Model file for the job. Use its own axes, mm. A direction names the side the tool comes from. Coordinates: 2 decimals unless noted, no trailing zeros. Order: outer loops, then holes, each group sorted by start corner. A loop starts at its lowest first (then second) coordinate and runs counter-clockwise, first axis right, second up.
from build123d import *
from OCP.BRepFilletAPI import BRepFilletAPI_MakeChamfer

# Parameters (mm, degrees)
ESQUISSE1_W           = 12
ESQUISSE1_H           = 12
BOSS_EXTRU_1_DEPTH    = 6.3
ESQUISSE2_R           = 3.4
BOSS_EXTRU_2_DEPTH    = 5
ESQUISSE5_R           = 1.8
BOSS_EXTRU_5_DEPTH    = 0.5
ESQUISSE3_R           = 3
BOSS_EXTRU_3_DEPTH    = 2.5
BOSS_EXTRU_6_START    = 2.5
BOSS_EXTRU_6_DEPTH    = 7
ESQUISSE4_W           = 1
ESQUISSE4_H           = 0.25
BOSS_EXTRU_4_DEPTH    = 3.8
CHANFREIN1_SIZE       = 0.5
CONG_1_R              = 1
CHANFREIN2_SIZE       = 0.3
CHANFREIN2_SIZE2      = 0.519615242
BOSS_EXTRU_7_START    = -1.2
BOSS_EXTRU_7_DEPTH    = 2
CONG_2_R              = 1
CONG_2_OF_SYM_TRIE1_R = 1


with BuildPart() as part:
    # Esquisse1 → Boss.-Extru.1 (new body)
    with BuildSketch(Plane.XY):
        Rectangle(ESQUISSE1_W, ESQUISSE1_H)
    extrude(amount=BOSS_EXTRU_1_DEPTH)

    # Esquisse2 → Boss.-Extru.2 (add)
    with BuildSketch(Plane.XY.offset(6.3)):
        Circle(ESQUISSE2_R)
    extrude(amount=BOSS_EXTRU_2_DEPTH)

    # Esquisse5 → Boss.-Extru.5 (add)
    with BuildSketch(Plane.XY.offset(11.3)):
        Circle(ESQUISSE5_R)
    extrude(amount=BOSS_EXTRU_5_DEPTH)

    # Esquisse3 → Boss.-Extru.3 (add)
    with BuildSketch(Plane.XY.offset(11.8)):
        Circle(ESQUISSE3_R)
    extrude(amount=BOSS_EXTRU_3_DEPTH)

    # Esquisse3<4> → Boss.-Extru.6 (add)
    with BuildSketch(Plane.XY.offset(11.8).offset(BOSS_EXTRU_6_START)):
        with BuildLine():
            Line((1.5, 0.994987437), (1.5, 2.598076211))
            ThreePointArc((1.5, 2.598076211), (-3, 0), (1.5, -2.598076211))
            Line((1.5, -2.598076211), (1.5, -0.994987437))
            ThreePointArc((1.5, -0.994987437), (-1.8, 0), (1.5, 0.994987437))
        make_face()
        with BuildLine():
            Line((1.5, -0.994987437), (1.5, 0.994987437))
            ThreePointArc((1.5, 0.994987437), (-1.8, 0), (1.5, -0.994987437))
        make_face()
    extrude(amount=BOSS_EXTRU_6_DEPTH)

    # Esquisse4 → Boss.-Extru.4 (add)
    with BuildSketch(Plane.XZ.offset(6)):
        with Locations((0, 3.5)):
            Rectangle(ESQUISSE4_W, ESQUISSE4_H)
        with Locations((2.35, 3.5)):
            Rectangle(ESQUISSE4_W, ESQUISSE4_H)
        with Locations((-2.35, 3.5)):
            Rectangle(ESQUISSE4_W, ESQUISSE4_H)
        with Locations((-2.35, 1)):
            Rectangle(ESQUISSE4_W, ESQUISSE4_H)
        with Locations((2.35, 1)):
            Rectangle(ESQUISSE4_W, ESQUISSE4_H)
    extrude(amount=BOSS_EXTRU_4_DEPTH)

    # Chanfrein1
    chanfrein1_edges = [part.edges().sort_by_distance(p)[0] for p in [
        (1.5, 0, 21.3),
        (-3, 0, 21.3),
    ]]
    chamfer(chanfrein1_edges, length=CHANFREIN1_SIZE)

    # Congé1
    cong_1_edges = [part.edges().sort_by_distance(p)[0] for p in [
        (6, -6, 3.15),
        (-6, -6, 3.15),
        (-6, 6, 3.15),
        (6, 6, 3.15),
    ]]
    fillet(cong_1_edges, radius=CONG_1_R)

    # Chanfrein2: one chamfer whose edges measure the first distance from different faces: ONE call of the kernel's chamfer builder (chamfer() names one face for all edges)
    chanfrein2_edges_1 = [part.edges().sort_by_distance(p)[0] for p in [
        (0.5, -6, 3.5),
    ]]
    chanfrein2_side_1 = [part.faces().sort_by_distance(p)[0] for p in [
        (0.5, -7.9, 3.5),
    ]]
    chanfrein2_edges_2 = [part.edges().sort_by_distance(p)[0] for p in [
        (-0.5, -6, 3.5),
    ]]
    chanfrein2_side_2 = [part.faces().sort_by_distance(p)[0] for p in [
        (-0.5, -7.9, 3.5),
    ]]
    chanfrein2_edges_3 = [part.edges().sort_by_distance(p)[0] for p in [
        (0.5, -9.8, 3.5),
        (-0.5, -9.8, 3.5),
    ]]
    chanfrein2_side_3 = [part.faces().sort_by_distance(p)[0] for p in [
        (0, -9.8, 3.5),
    ]]
    chanfrein2_edges_4 = [part.edges().sort_by_distance(p)[0] for p in [
        (2.85, -6, 3.5),
    ]]
    chanfrein2_side_4 = [part.faces().sort_by_distance(p)[0] for p in [
        (2.85, -7.9, 3.5),
    ]]
    chanfrein2_edges_5 = [part.edges().sort_by_distance(p)[0] for p in [
        (1.85, -6, 3.5),
    ]]
    chanfrein2_side_5 = [part.faces().sort_by_distance(p)[0] for p in [
        (1.85, -7.9, 3.5),
    ]]
    chanfrein2_edges_6 = [part.edges().sort_by_distance(p)[0] for p in [
        (2.85, -9.8, 3.5),
        (1.85, -9.8, 3.5),
    ]]
    chanfrein2_side_6 = [part.faces().sort_by_distance(p)[0] for p in [
        (2.35, -9.8, 3.5),
    ]]
    chanfrein2_edges_7 = [part.edges().sort_by_distance(p)[0] for p in [
        (-1.85, -6, 3.5),
    ]]
    chanfrein2_side_7 = [part.faces().sort_by_distance(p)[0] for p in [
        (-1.85, -7.9, 3.5),
    ]]
    chanfrein2_edges_8 = [part.edges().sort_by_distance(p)[0] for p in [
        (-2.85, -6, 3.5),
    ]]
    chanfrein2_side_8 = [part.faces().sort_by_distance(p)[0] for p in [
        (-2.85, -7.9, 3.5),
    ]]
    chanfrein2_edges_9 = [part.edges().sort_by_distance(p)[0] for p in [
        (-1.85, -9.8, 3.5),
        (-2.85, -9.8, 3.5),
    ]]
    chanfrein2_side_9 = [part.faces().sort_by_distance(p)[0] for p in [
        (-2.35, -9.8, 3.5),
    ]]
    chanfrein2_edges_10 = [part.edges().sort_by_distance(p)[0] for p in [
        (-1.85, -6, 1),
    ]]
    chanfrein2_side_10 = [part.faces().sort_by_distance(p)[0] for p in [
        (-1.85, -7.9, 1),
    ]]
    chanfrein2_edges_11 = [part.edges().sort_by_distance(p)[0] for p in [
        (-2.85, -6, 1),
    ]]
    chanfrein2_side_11 = [part.faces().sort_by_distance(p)[0] for p in [
        (-2.85, -7.9, 1),
    ]]
    chanfrein2_edges_12 = [part.edges().sort_by_distance(p)[0] for p in [
        (-1.85, -9.8, 1),
        (-2.85, -9.8, 1),
    ]]
    chanfrein2_side_12 = [part.faces().sort_by_distance(p)[0] for p in [
        (-2.35, -9.8, 1),
    ]]
    chanfrein2_edges_13 = [part.edges().sort_by_distance(p)[0] for p in [
        (2.85, -6, 1),
    ]]
    chanfrein2_side_13 = [part.faces().sort_by_distance(p)[0] for p in [
        (2.85, -7.9, 1),
    ]]
    chanfrein2_edges_14 = [part.edges().sort_by_distance(p)[0] for p in [
        (1.85, -6, 1),
    ]]
    chanfrein2_side_14 = [part.faces().sort_by_distance(p)[0] for p in [
        (1.85, -7.9, 1),
    ]]
    chanfrein2_edges_15 = [part.edges().sort_by_distance(p)[0] for p in [
        (2.85, -9.8, 1),
        (1.85, -9.8, 1),
    ]]
    chanfrein2_side_15 = [part.faces().sort_by_distance(p)[0] for p in [
        (2.35, -9.8, 1),
    ]]
    chanfrein2 = BRepFilletAPI_MakeChamfer(part.part.solid().wrapped)
    for e in chanfrein2_edges_1:
        chanfrein2.Add(CHANFREIN2_SIZE, CHANFREIN2_SIZE2, e.wrapped, chanfrein2_side_1[0].wrapped)  # the first distance lies on this face
    for e in chanfrein2_edges_2:
        chanfrein2.Add(CHANFREIN2_SIZE, CHANFREIN2_SIZE2, e.wrapped, chanfrein2_side_2[0].wrapped)  # the first distance lies on this face
    for e in chanfrein2_edges_3:
        chanfrein2.Add(CHANFREIN2_SIZE, CHANFREIN2_SIZE2, e.wrapped, chanfrein2_side_3[0].wrapped)  # the first distance lies on this face
    for e in chanfrein2_edges_4:
        chanfrein2.Add(CHANFREIN2_SIZE, CHANFREIN2_SIZE2, e.wrapped, chanfrein2_side_4[0].wrapped)  # the first distance lies on this face
    for e in chanfrein2_edges_5:
        chanfrein2.Add(CHANFREIN2_SIZE, CHANFREIN2_SIZE2, e.wrapped, chanfrein2_side_5[0].wrapped)  # the first distance lies on this face
    for e in chanfrein2_edges_6:
        chanfrein2.Add(CHANFREIN2_SIZE, CHANFREIN2_SIZE2, e.wrapped, chanfrein2_side_6[0].wrapped)  # the first distance lies on this face
    for e in chanfrein2_edges_7:
        chanfrein2.Add(CHANFREIN2_SIZE, CHANFREIN2_SIZE2, e.wrapped, chanfrein2_side_7[0].wrapped)  # the first distance lies on this face
    for e in chanfrein2_edges_8:
        chanfrein2.Add(CHANFREIN2_SIZE, CHANFREIN2_SIZE2, e.wrapped, chanfrein2_side_8[0].wrapped)  # the first distance lies on this face
    for e in chanfrein2_edges_9:
        chanfrein2.Add(CHANFREIN2_SIZE, CHANFREIN2_SIZE2, e.wrapped, chanfrein2_side_9[0].wrapped)  # the first distance lies on this face
    for e in chanfrein2_edges_10:
        chanfrein2.Add(CHANFREIN2_SIZE, CHANFREIN2_SIZE2, e.wrapped, chanfrein2_side_10[0].wrapped)  # the first distance lies on this face
    for e in chanfrein2_edges_11:
        chanfrein2.Add(CHANFREIN2_SIZE, CHANFREIN2_SIZE2, e.wrapped, chanfrein2_side_11[0].wrapped)  # the first distance lies on this face
    for e in chanfrein2_edges_12:
        chanfrein2.Add(CHANFREIN2_SIZE, CHANFREIN2_SIZE2, e.wrapped, chanfrein2_side_12[0].wrapped)  # the first distance lies on this face
    for e in chanfrein2_edges_13:
        chanfrein2.Add(CHANFREIN2_SIZE, CHANFREIN2_SIZE2, e.wrapped, chanfrein2_side_13[0].wrapped)  # the first distance lies on this face
    for e in chanfrein2_edges_14:
        chanfrein2.Add(CHANFREIN2_SIZE, CHANFREIN2_SIZE2, e.wrapped, chanfrein2_side_14[0].wrapped)  # the first distance lies on this face
    for e in chanfrein2_edges_15:
        chanfrein2.Add(CHANFREIN2_SIZE, CHANFREIN2_SIZE2, e.wrapped, chanfrein2_side_15[0].wrapped)  # the first distance lies on this face
    add(Compound.cast(chanfrein2.Shape()), mode=Mode.REPLACE)

    # Esquisse6 → Boss.-Extru.7 (add)
    with BuildSketch(Plane(origin=(0, 0, 0), x_dir=(-1, 0, 0), z_dir=(0, 0, -1)).offset(BOSS_EXTRU_7_START)):
        with BuildLine():
            Line((-6, -4.090148625), (-6.15, -4.090148625))
            ThreePointArc((-6.15, -4.090148625), (-6.432842712, -4.207305912), (-6.55, -4.490148625))
            Line((-6.55, -4.490148625), (-6.55, -7.432968948))
            ThreePointArc((-6.55, -7.432968948), (-6.563629669, -7.536496566), (-6.603589838, -7.632968948))
            Line((-6.603589838, -7.632968948), (-7.006574145, -8.330958241))
            ThreePointArc((-7.006574145, -8.330958241), (-7.059189603, -8.55886083), (-6.975368285, -8.777222831))
            Line((-6.975368285, -8.777222831), (-5.969546479, -10.064616035))
            Line((-5.969546479, -10.064616035), (-5.614941639, -9.787568371))
            Line((-5.614941639, -9.787568371), (-6.433892437, -8.739359151))
            ThreePointArc((-6.433892437, -8.739359151), (-6.517713755, -8.52099715), (-6.465098297, -8.293094561))
            Line((-6.465098297, -8.293094561), (-6.153589838, -7.753546084))
            ThreePointArc((-6.153589838, -7.753546084), (-6.113629669, -7.657073702), (-6.1, -7.553546084))
            Line((-6.1, -7.553546084), (-6.1, -4.540148625))
            Line((-6.1, -4.540148625), (-6, -4.540148625))
            Line((-6, -4.540148625), (-6, -4.090148625))
        make_face()
    boss_extru_7 = extrude(amount=-BOSS_EXTRU_7_DEPTH)

    # Congé2
    cong_2_edges = [part.edges().sort_by_distance(p)[0] for p in [
        (5.792244059, -9.926092203, 1.2),
        (5.792244059, -9.926092203, 3.2),
    ]]
    fillet(cong_2_edges, radius=CONG_2_R - 0.0001)  # a hair under: the kernel refuses the full size

    # Symétrie1: Boss.-Extru.7 across plane
    add(boss_extru_7.mirror(Plane(origin=(0, 0, 0), x_dir=(0, 0, 1), z_dir=(1, 0, 0))))

    # Congé2 of Symétrie1
    cong_2_of_sym_trie1_edges = [part.edges().sort_by_distance(p)[0] for p in [
        (-5.792244059, -9.926092203, 1.2),
        (-5.792244059, -9.926092203, 3.2),
    ]]
    fillet(cong_2_of_sym_trie1_edges, radius=CONG_2_OF_SYM_TRIE1_R - 0.0001)  # a hair under: the kernel refuses the full size


solid = part.part
Q1. Cut at B-B, the plane y = 0. List the corners of the cut face in (x, z), plus the area to 3 significant figures.
Established:
outline: (-6, 0) - (6, 0) - (6, 6.3) - (3.4, 6.3) - (3.4, 11.3) - (1.8, 11.3) - (1.8, 11.8) - (3, 11.8) - (3, 14.3) - (1.5, 14.3) - (1.5, 20.8) - (1, 21.3) - (-2.5, 21.3) - (-3, 20.8) - (-3, 11.8) - (-1.8, 11.8) - (-1.8, 11.3) - (-3.4, 11.3) - (-3.4, 6.3) - (-6, 6.3) - close
area: 158 mm2
Q2. Mould opens along X. For faces 4 (the face through (0, -2, 11.8)), 5 (the face through (5.699, -5.715, 3.194)), 6 (the face through (-5.715, 5.699, 3.194)) say: pulls with the +X half, pulls with the -X half, needs draft (parallel to the pull), parting line crosses it, or undercut.
Established:
face 4: needs draft
face 5: undercut
face 6: pulls with the -X half
Q3. Cut at D-D, the plane y = 4.75. List the corners of the cut face in (x, z).
Established:
outline: (-6, 0) - (6, 0) - (6, 6.3) - (-6, 6.3) - close
Q4. Drop flat-ended pins along their axis: P1, Ø4, axis at y = 4, z = 5.5, coming from the -X side; P2, Ø1, axis at x = 2, y = -8.5, coming from the +Z side (3 decimals); P3, Ø1, axis at y = 0, z = 7.5, coming from the +X side; P4, Ø1, axis at x = -4, z = 6.5, coming from the +Y side. Give the stop position or say it passes through.
Established:
P1: stops at x = -6
P2: stops at z = 3.625
P3: stops at x = 3.4
P4: stops at y = 6
Q5. Probe line 1 (X direction, y = -0.75, z = 6.25); line 2 (Z direction, x = -5.25, y = -4.75). List the from-to ranges inside material, lowest first.
Established:
line 1: x = -6 to 6
line 2: z = 0 to 6.3
Q6. Which spindle directions (+Z, -Z, +X, -X, +Y, -Y) get a long thin tool onto all of the face, cutting with end or side? Do faces 1 (the face through (-5.97, -9.69, 1.49)), 2 (the face through (-2.4, -7.9, 3.375)), 3 (the face through (-6.3, -6.6, 1.2)). Say none if no direction does.
Established:
face 1: -Z, -Y
face 2: +X, -X, -Y
face 3: -Z, -X, +Y, -Y
Q7. Cut at C-C, the plane z = 19.25. List the corners of the cut face in (x, y).
Established:
outline: (1.5, -2.6) - (1.5, 2.6) arc R3 ccw (long way) to start
Q8. Cut at A-A, the plane z = 4. List the corners of the cut face in (x, y), plus the area to 3 significant figures.
Established:
outline: (-6, -5) arc R1 ccw to (-5, -6) - (5, -6) arc R1 ccw to (6, -5) - (6, 5) arc R1 ccw to (5, 6) - (-5, 6) arc R1 ccw to (-6, 5) - close
area: 143 mm2
